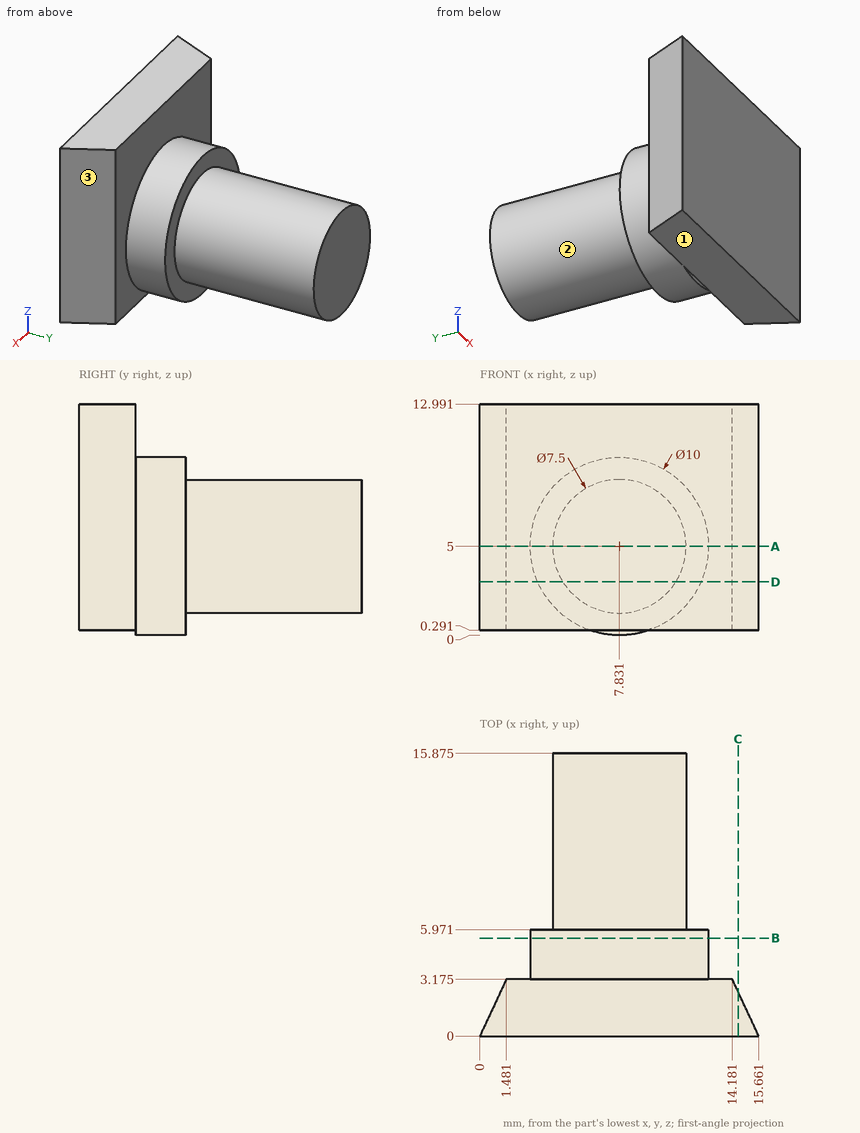
Verification items for this drawing (mm, ordinates from the low corner). A direction names the side the tool comes from. Round coordinates to 2 decimals unless told otherwise and drop trailing zeros. Order: outer loops, then holes, each group sorted by start corner. A loop starts at its lowest first (then second) coordinate and runs counter-clockwise, first axis right, second up. Notation, with made-up numbers: M 70,59 L 122,59 A18 cw 122,77 Z; hole C 3,-22 d11. An arc over 180 degrees is marked long. Answer in a Markdown table with one row per item. Add a question column.
Item 1: Sectioned sample at C-C, the plane x = 14.5. Enter the section's corners in (y, z).
Item 2: Set-up check for the marked faces 1, 2 and 3: record each of +Z, -Z, +X, -X, +Y, -Y from which the full face is reachable in a straight line by a thin tool's end or side.
Item 3: Sectioned sample at D-D, the plane z = 3. Enter the section's corners in (x, y) (1 decimal).
Item 4: Sectioned sample at A-A, the plane z = 5. Enter the section's corners in (x, y) (1 decimal), plus the area to 3 significant figures.
Item 5: Depth check by flat-ended pin: pin 1 Ø3 at (x, z) = (2, 9) entering from +Y (3 decimals); pin 2 Ø5 at (x, y) = (4, 12) entering from +Z (1 decimal); pin 3 Ø4 at (x, y) = (14, 5.5) entering from +Z. Enter the tip coordinate at first touch or a pass-through.
Item 6: Material ranges on L1, parallel to Y at x = 1.75, z = 3.25 (1 decimal); L2, parallel to Z at x = 1.25, y = 2.5; L3, parallel to Y at x = 3.25, z = 4.5, recorded low to high. Write a range as [from, to].
Item 7: Sectioned sample at B-B, the plane y = 5.5. Enter the section's corners in (x, z).
Filled in:
| question | item | result |
|---|---|---|
| 1 | outline | M 0,0.29 L 2.49,0.29 L 2.49,12.99 L 0,12.99 Z |
| 2 | face 1 | -Z, +X, -X, -Y |
| 2 | face 2 | +Y |
| 2 | face 3 | +Z, -Z, +X, +Y |
| 3 | outline | M 0,0 L 15.7,0 L 14.2,3.2 L 12.4,3.2 L 12.4,6 L 11,6 L 11,15.9 L 4.7,15.9 L 4.7,6 L 3.2,6 L 3.2,3.2 L 1.5,3.2 Z |
| 4 | outline | M 0,0 L 15.7,0 L 14.2,3.2 L 12.8,3.2 L 12.8,6 L 11.6,6 L 11.6,15.9 L 4.1,15.9 L 4.1,6 L 2.8,6 L 2.8,3.2 L 1.5,3.2 Z |
| 4 | area | 147 mm² |
| 5 | pin 1 | stops at y = 3.175 |
| 5 | pin 2 | stops at z = 8.5 |
| 5 | pin 3 | stops at z = 7.76 |
| 6 | L1 | y = [0, 3.2] |
| 6 | L2 | z = [0.29, 12.99] |
| 6 | L3 | y = [0, 5.97] |
| 7 | outline | C 7.83,5 d10 |
